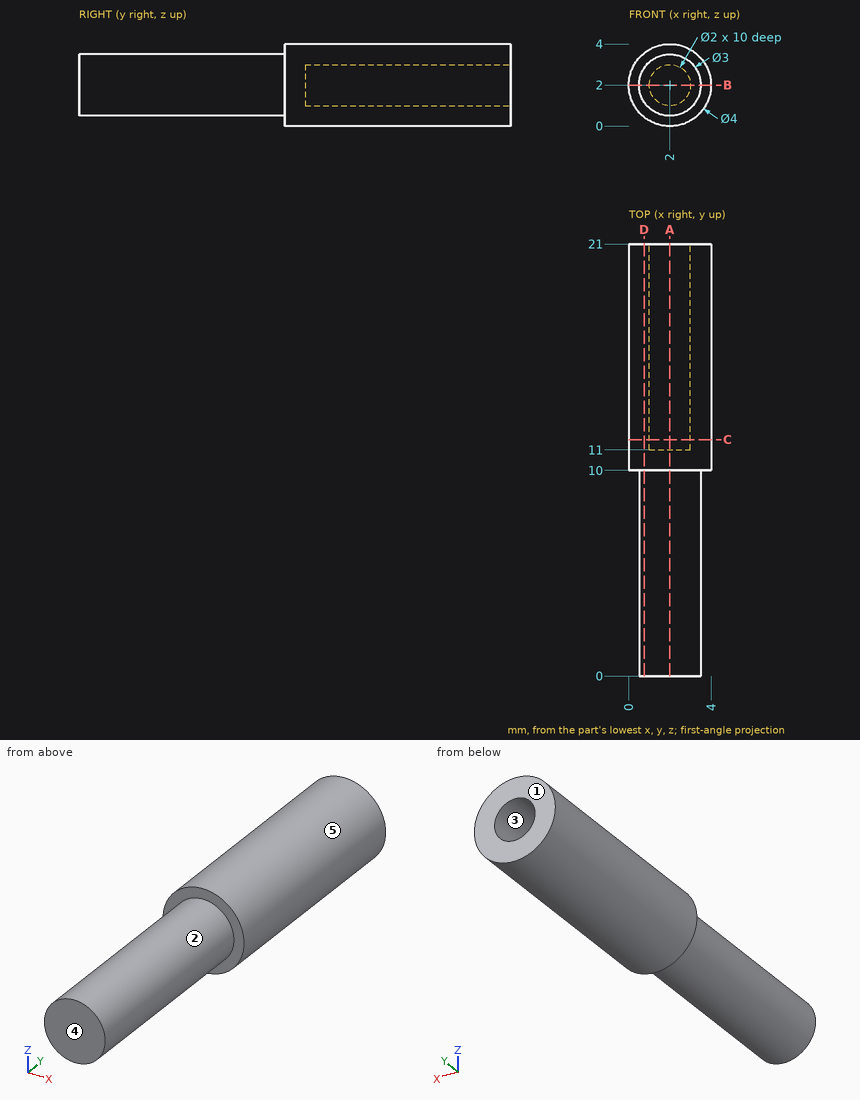
Geometry check sheet. Reference: drawing and pictorial views, mm from the part's lowest x, y, z. A direction names the side the tool comes from. Give positions to 0.01 mm unless a question says otherwise; leave off trailing zeros. Write each loop counter-clockwise with the first axis right and the second up, starting at its lowest first coordinate (ties: lowest second). Pieces come first, ordered by that corner, then holes. Notation, with made-up numbers: (1, 64.25) -> (5, 64.25) arc R20 cw to (5, 89.25) -> close; hole circle Ø5 at (-24, 44). An arc over 180 degrees is marked (long way). One line per item, written item: value. Start each with the question number.
Item 1: Section check B-B on z = 2. Record the cut outline in (x, y).
Item 2: Draft check along X on the marked faces 3, 4 and 5. Enter one of: +X half, -X half, draft (parallel to the pull), parting line (faces both ways), or undercut.
Item 3: Tool access check on the marked faces 1 and 2. Record the directions out of +Z, -Z, +X, -X, +Y, -Y that give a thin tool (end or side, any length) a straight path to the whole face; none if there is none.
Item 4: Section check C-C on y = 11.5. Record the cut outline in (x, z).
Item 5: Section check A-A on x = 2. Record the cut outline in (y, z).
Item 6: Material ranges on probe 1 along Z at (x, y) = (2, 16); probe 2 along Y at (x, z) = (2.7, 2.25); probe 3 along Y at (x, z) = (3.35, 1.25), recorded low to high. Write a range as from..to.
Item 7: Section check D-D on x = 0.75. Record the cut outline in (y, z), then the cut area to 3 significant figures.
Item 8: Gauge pin test, flat ends, axial feed: pin 1 (1 mm diameter, centred on x = 0.5, y = 15.5, fed in from +Z); pin 2 (1.5 mm diameter, centred on x = 1.5, y = 7.5, fed in from -Z); pin 3 (1 mm diameter, centred on y = 7.5, z = 2.5, fed in from +X). Record the tip position at first contact, or that the pin passes through.
Results list:
1. outline: (0, 10) -> (0.5, 10) -> (0.5, 0) -> (3.5, 0) -> (3.5, 10) -> (4, 10) -> (4, 21) -> (3, 21) -> (3, 11) -> (1, 11) -> (1, 21) -> (0, 21) -> close
2. face 3: undercut
2. face 4: draft
2. face 5: parting line
3. face 1: +Z, -Z, +X, -X, +Y
3. face 2: -Y
4. outline: circle Ø4 at (2, 2); hole circle Ø2 at (2, 2)
5. outline: (0, 0.5) -> (10, 0.5) -> (10, 0) -> (21, 0) -> (21, 1) -> (11, 1) -> (11, 3) -> (21, 3) -> (21, 4) -> (10, 4) -> (10, 3.5) -> (0, 3.5) -> close
6. probe 1: 0..1, 3..4
6. probe 2: 0..11
6. probe 3: 10..21
7. outline: (0, 1.17) -> (10, 1.17) -> (10, 0.44) -> (21, 0.44) -> (21, 3.56) -> (10, 3.56) -> (10, 2.83) -> (0, 2.83) -> close
7. area: 50.9 mm²
8. pin 1: z = 3.73
8. pin 2: z = 0.5
8. pin 3: x = 3.5
